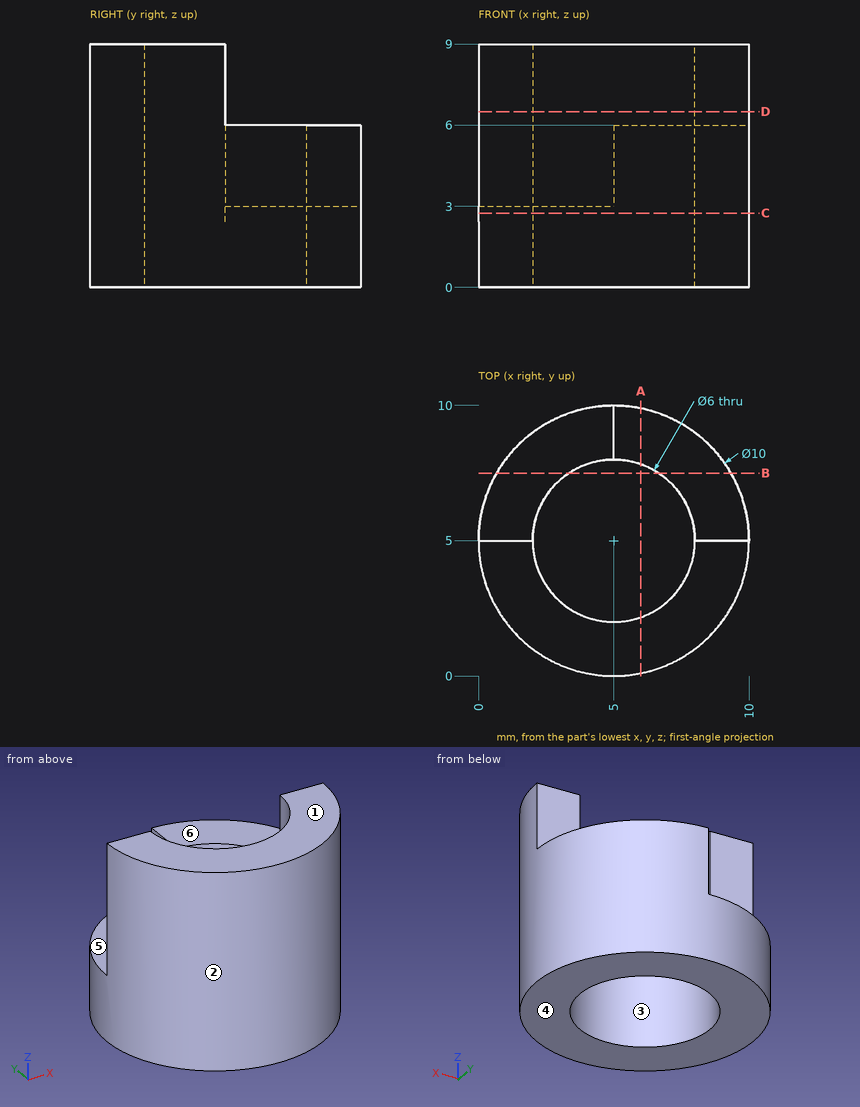
Input: dimensioned drawing with shaded views. Units: mm. Origin: part minimum x, y, z. A direction names the side the tool comes from. Round coordinates to 2 decimals unless told otherwise and drop trailing zeros. Loops run counter-clockwise (first coordinate to the right, second up) from the corner with the lowest first, then second, coordinate; pieces in that order, holes last. Notation, with made-up numbers: M 0,-21 L 57,-21 A15 cw 57,7 Z; hole C 17,46.5 d9. An arc over 180 degrees is marked long. One line per question, with ' | ' between items.
(1) Cut plane B-B on y = 7.5. Return the cut outline in (x, z).
Check result:
outline: M 0.67,0 L 3.34,0 L 3.34,3 L 0.67,3 Z; M 6.66,0 L 9.33,0 L 9.33,6 L 6.66,6 Z
(2) Cut plane C-C on z = 2.75. Return the cut outline in (x, y), plus the area to 3 significant figures.
Check result:
outline: C 5,5 d10; hole C 5,5 d6 | area: 50.3 mm2
(3) Pull-direction query (Y, two-part tool) for the marked faces 1, 2 and 3; classes: +Y half, -Y half, draft (parallel to the pull), parting line (faces both ways), or undercut.
Check result:
face 1: draft | face 2: parting line | face 3: undercut
(4) Contact query for flat-ended pins moving along their axis: P1, Ø1, axis at y = 9, z = 4, coming from the -X side; P2, Ø1, axis at x = 7.5, y = 7, coming from the +Z side; P3, Ø1.5, axis at x = 2, y = 6.5, coming from the +Z side. Output: stop coordinate, or through.
Check result:
P1: stops at x = 5 | P2: stops at z = 6 | P3: stops at z = 3
(5) Material intervals for line 1 along Y through (x, z) = (5, 2); line 2 along Y through (x, z) = (9, 0.5); line 3 along X through (y, z) = (4.25, 3), sorted ascending. Write a range as from..to.
Check result:
line 1: y = 0..2, 8..10 | line 2: y = 2..8 | line 3: x = 0.06..2.1, 7.9..9.94
(6) Cut plane A-A on x = 6. Return the cut outline in (y, z), plus the area to 3 significant figures.
Check result:
outline: M 0.1,0 L 2.17,0 L 2.17,9 L 0.1,9 Z; M 7.83,0 L 9.9,0 L 9.9,6 L 7.83,6 Z | area: 31.1 mm2
(7) Access query for the marked faces 4, 5 and 6. Directions: +Z, -Z, +X, -X, +Y, -Y. A direction counts if a zero-diameter tool reaches every point of the face in a straight line with its end or side. Return the directions, or none.
Check result:
face 4: -Z, +X, -X, +Y, -Y | face 5: +Z, -X, +Y | face 6: +Z, +X, -X, +Y
(8) Cut plane D-D on z = 6.5. Return the cut outline in (x, y).
Check result:
outline: M 0,5 A5 ccw 10,5 L 8,5 A3 cw 2,5 Z
